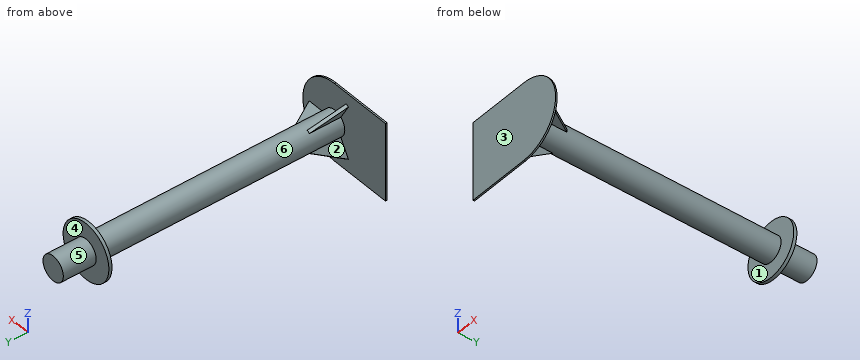
```python
from build123d import *

# Parameters (mm, degrees)
EXTRUDE_1_DEPTH          = 5
SKETCH_2_R               = 40
EXTRUDE_2_DEPTH          = 900
SKETCH_3_R               = 90
EXTRUDE_3_DEPTH          = 10
EXTRUDE_6_DEPTH          = 5
PATTERN_CIRCULAR_1_COUNT = 3


with BuildPart() as part:
    # 草图1 → 凸台-拉伸1 (new body)
    with BuildSketch(Plane(origin=(0, 0, 0), x_dir=(1, 0, 0), z_dir=(0, 1, 0))):
        with BuildLine():
            Line((-119.91416309, -125), (-119.91416309, 125))
            Line((-119.91416309, 125), (80.08583691, 125))
            ThreePointArc((80.08583691, 125), (205.08583691, 0), (80.08583691, -125))
            Line((80.08583691, -125), (-119.91416309, -125))
        make_face()
    extrude(amount=EXTRUDE_1_DEPTH)

    # 草图2 → 凸台-拉伸2 (add)
    with BuildSketch(Plane(origin=(0, 5, 0), x_dir=(1, 0, 0), z_dir=(0, 1, 0))):
        with Locations(Location((80.08583691, 0, 0), (0, 0, 90))):
            Circle(SKETCH_2_R)
    extrude(amount=EXTRUDE_2_DEPTH)

    # 草图3 → 凸台-拉伸3 (add)
    with BuildSketch(Plane(origin=(0, 790, 0), x_dir=(-1, 0, 0), z_dir=(0, -1, 0))):
        with Locations(Location((-80.08583691, 0, 0), (0, 0, 90))):
            Circle(SKETCH_3_R)
    extrude(amount=-EXTRUDE_3_DEPTH)

    # 草图5 → 凸台-拉伸6 (add, symmetric)
    with BuildSketch(Plane.XY):
        Polygon((108.365396312, 5), (120.08583691, 5), (120.08583691, 105), (108.365396312, 124.534067663), align=None)
        Polygon((120.08583691, 5), (180.08583691, 5), (120.08583691, 105), align=None)
    extrude_6 = extrude(amount=EXTRUDE_6_DEPTH, both=True)

    # 阵列(圆周)1: 凸台-拉伸6 ×3 about axis
    pattern_circular_1_axis = Axis((80.08583691, 0, 0), (0, 1, 0))
    for i in range(1, PATTERN_CIRCULAR_1_COUNT):
        add(extrude_6.rotate(pattern_circular_1_axis, i * 360 / PATTERN_CIRCULAR_1_COUNT))


solid = part.part
```
Read the model definition and answer for the solid it produces. Units are mm, in the model's axes. Face numbers are marked on the shaded views. A direction names the side the tool comes from. Coordinates: 2 decimals unless noted, no trailing zeros. Write each loop counter-clockwise with the first axis right and the second up, starting at its lowest first coordinate (ties: lowest second). Pieces come first, ordered by that corner, then holes. Notation, with made-up numbers: (-7.75, 60) -> (35.25, 60) arc R13 ccw to (35.25, 82) -> close; hole circle Ø10 at (88, 71.25). An arc over 180 degrees is marked (long way). Write item = value, one per line.
(1) Which of the six approach directions +Z, -Z, +X, -X, +Y, -Y give full straight-line access (tool end or side, diameter ignored) to the marked faces 1, 2 and 3?
From the geometry:
face_1 = none
face_2 = -X
face_3 = +Z, -Z, +X, -X, -Y
(2) Section A-A on z = 74.5 is taken. Write down the section's boundary in (x, y).
From the geometry:
outline = (-119.91, 0) -> (180.46, 0) -> (180.46, 5) -> (42.85, 5) -> (42.85, 33.1) -> (31.3, 23.48) -> (31.3, 5) -> (-119.91, 5) -> close; (29.59, 790) -> (130.58, 790) -> (130.58, 800) -> (29.59, 800) -> close
(3) Straight lines are drawn through the part: L1, parallel to Y at x = 110, z = -28.5; L2, parallel to Y at x = -23, z = -17.5; L3, parallel to Z at x = 107, y = 142.5. For each, find the intervals that lie inside material, in ascending order. Write a range as from..to.
From the geometry:
L1 = 0..5, 790..800
L2 = 0..5
L3 = -29.59..29.59
(4) Section D-D on y = 56 is taken. Write down the section's boundary in (x, z), plus the area to 3 significant figures.
From the geometry:
outline = (41.06, -57.6) -> (49.72, -62.6) -> (64.57, -36.87) arc R40 ccw to (119.77, -5) -> (149.49, -5) -> (149.49, 5) -> (119.77, 5) arc R40 ccw to (64.57, 36.87) -> (49.72, 62.6) -> (41.06, 57.6) -> (55.91, 31.87) arc R40 ccw to (55.91, -31.87) -> close
area = 5,910 mm2
(5) For a pull along Y with two mould halves and no side action, classify the marked faces 4, 5 and 6 as +Y half, -Y half, draft (parallel to the pull), parting line (faces both ways), or undercut.
From the geometry:
face_4 = +Y half
face_5 = draft
face_6 = undercut
(6) Given pin 1 Ø12 at (y, z) = (788, -19) entering from +X; pin 2 Ø1.5 at (y, z) = (475, -32) entering from -X, each flat-ended and moving along its own axis, determine where each tip first touches the part or whether it passes through.
From the geometry:
pin_1 = 169.09
pin_2 = 55.12
(7) Section C-C on x = -99 is taken. Write down the section's boundary in (y, z).
From the geometry:
outline = (0, -125) -> (5, -125) -> (5, 125) -> (0, 125) -> close
(8) Section B-B on y = 359.5 is taken. Write down the section's boundary in (x, z).
From the geometry:
outline = circle Ø80 at (80.09, 0)
